The drawing under review shows one solid part. Ordinate dimensions are in mm from its lowest x, y, z. Coordinates: 2 decimals unless noted, no trailing zeros. Order: outer loops, then holes, each group sorted by start corner. A loop starts at its lowest first (then second) coordinate and runs counter-clockwise, first axis right, second up.
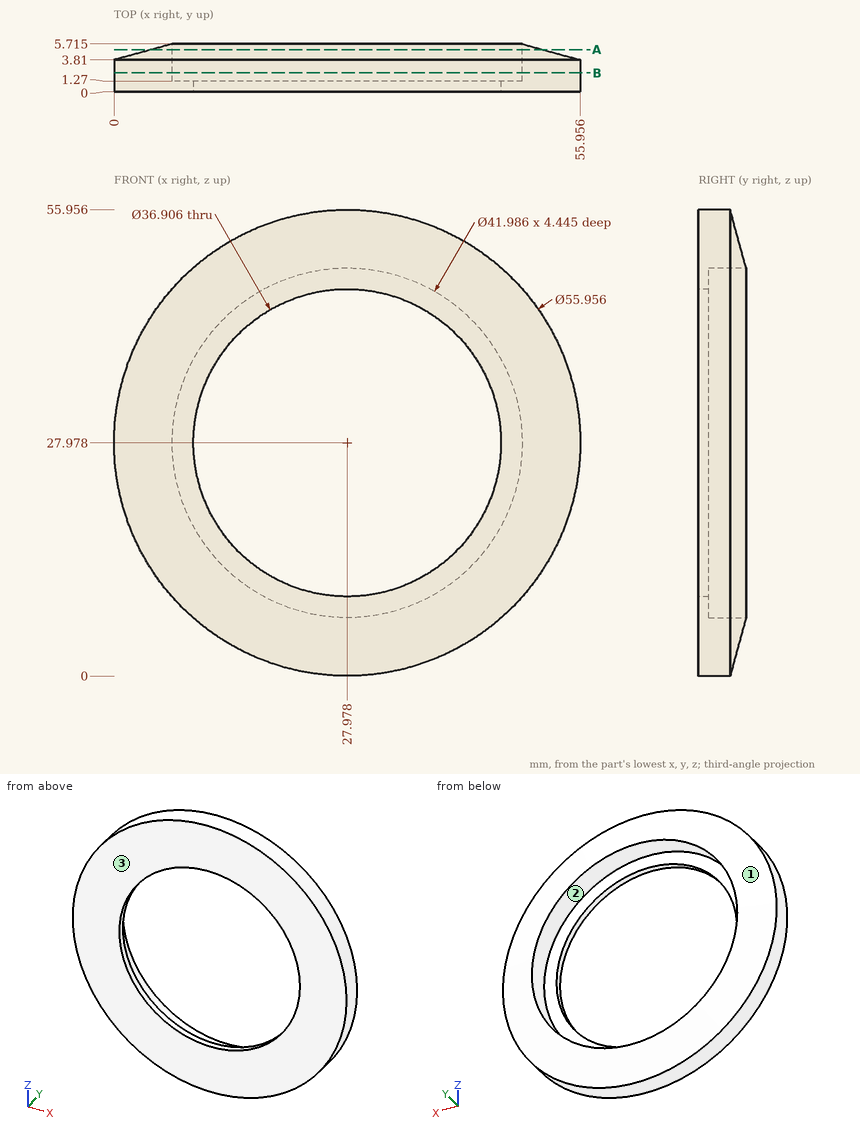
(1) Draft analysis for pull direction X (two halves, no side actions). For the marked faces 1, 2 and 3, state which applies: released by +X, released by -X, zero draft, split by the parting line, or undercut.
A:
face 1: split by the parting line
face 2: undercut
face 3: zero draft
(2) We need section A-A, the plane y = 5.05. Write out the cut boundary in (x, z), and give its area (3 significant figures).
A:
outline: circle Ø46.86 at (27.98, 27.98); hole circle Ø41.99 at (27.98, 27.98)
area: 340 mm2
(3) We need section B-B, the plane y = 2.25. Write out the cut boundary in (x, z), and give its area (3 significant figures).
A:
outline: circle Ø55.96 at (27.98, 27.98); hole circle Ø41.99 at (27.98, 27.98)
area: 1,070 mm2
(4) For pin 1 Ø21 at (x, z) = (37.5, 31.5) entering from +Y; pin 2 Ø8 at (x, z) = (28.5, 41) entering from -Y; pin 3 Ø2 at (x, y) = (7, 4) entering from -Z; pin 4 Ø3 at (y, z) = (4.5, 34.5) entering from -X, all flat-tipped, find the tip position at first contact; note any pin that passes through.
A:
pin 1: stops at y = 1.27
pin 2: passes through
pin 3: stops at z = 8.41
pin 4: stops at x = 0.49
(5) Wall thickness on probe 1 along Y at (x, z) = (26.5, 8.5); probe 2 along X at (y, z) = (1.4, 14) (1 decimal); probe 3 along X at (y, z) = (3, 28) (1 decimal): over which ranges is each line inside the solid? List them lowest first.
A:
probe 1: y = 0 to 1.27
probe 2: x = 3.7 to 12.3, 43.6 to 52.2
probe 3: x = 0 to 7, 49 to 56
